Build history of the part. All positions in model axes, mm. A direction names the side the tool comes from. Round coordinates to 2 decimals unless told otherwise and drop trailing zeros. Loops run counter-clockwise (first coordinate to the right, second up) from the corner with the lowest first, then second, coordinate; pieces in that order, holes last.
from build123d import *

# Parameters (mm, degrees)
F0_W     = 88.9
F0_H     = 165.1
F1_DEPTH = 6.35
F2_DEPTH = 25.4
F3_DEPTH = 50.8
F4_SIZE2 = 7.3323484187
F4_SIZE  = 12.7
F5_R     = 6.34999
F6_SIZE2 = 7.3323484187
F6_SIZE  = 12.7
F7_SIZE2 = 7.3323484187
F7_SIZE  = 12.7


# Not quite as in the source:
# - a fillet or chamfer is up to 0.001 mm smaller than in the source, because OpenCascade refuses the exact size


with BuildPart() as f1:
    # F0 (on Top) → F1 (new body)
    with BuildSketch(Plane.XY):
        Rectangle(F0_W, F0_H)
        Polygon((-38.1, 38.1), (-38.1, 76.2), (0, 76.2), (38.1, 76.2), (38.1, -38.1), (38.1, -76.2), (0, -76.2), (-38.1, -76.2), align=None, mode=Mode.SUBTRACT)
    extrude(amount=F1_DEPTH)

    # F0 (on Top) → F2 (join)
    with BuildSketch(Plane.XY):
        with BuildLine():
            Line((38.1, 76.2), (0, 76.2))
            Line((0, 76.2), (0, 50.8))
            ThreePointArc((0, 50.8), (-3.7197438789, 41.8197438789), (-12.7, 38.1))
            Line((-12.7, 38.1), (-38.1, 38.1))
            Line((-38.1, 38.1), (-38.1, -76.2))
            Line((-38.1, -76.2), (0, -76.2))
            Line((0, -76.2), (0, -50.8))
            ThreePointArc((0, -50.8), (3.7197438789, -41.8197438789), (12.7, -38.1))
            Line((12.7, -38.1), (38.1, -38.1))
            Line((38.1, -38.1), (38.1, 76.2))
        make_face()
    extrude(amount=F2_DEPTH)

    # F0 (on Top) → F3 (join)
    with BuildSketch(Plane.XY):
        with BuildLine():
            Line((0, 76.2), (-38.1, 76.2))
            Line((-38.1, 76.2), (-38.1, 38.1))
            Line((-38.1, 38.1), (-12.7, 38.1))
            ThreePointArc((-12.7, 38.1), (-3.7197438789, 41.8197438789), (0, 50.8))
            Line((0, 50.8), (0, 76.2))
        make_face()
        with BuildLine():
            Line((38.1, -76.2), (38.1, -38.1))
            Line((38.1, -38.1), (12.7, -38.1))
            ThreePointArc((12.7, -38.1), (3.7197438789, -41.8197438789), (0, -50.8))
            Line((0, -50.8), (0, -76.2))
            Line((0, -76.2), (38.1, -76.2))
        make_face()
    extrude(amount=F3_DEPTH)

    # F4
    f4_edges = [f1.edges().sort_by_distance(p)[0] for p in [
        (-38.1, -19.05, 25.4),
        (-19.05, -76.2, 25.4),
        (38.1, 19.05, 25.4),
        (19.05, 76.2, 25.4),
    ]]
    f4_side = f1.faces().sort_by_distance((0, 0, 25.4))[0]
    chamfer(f4_edges, length=F4_SIZE, length2=F4_SIZE2, reference=f4_side)

    # F5 (radius 6.35 in the source; OpenCascade refuses exactly that, so slightly less here)
    f5_edges = [f1.edges().sort_by_distance(p)[0] for p in [
        (44.45, 0, 6.35),
        (0, -82.55, 6.35),
        (-44.45, 0, 6.35),
        (0, 82.55, 6.35),
    ]]
    fillet(f5_edges, radius=F5_R)

    # F6
    f6_edges = [f1.edges().sort_by_distance(p)[0] for p in [
        (-19.05, 76.2, 50.8),
        (-38.1, 57.15, 50.8),
    ]]
    chamfer(f6_edges, length=F6_SIZE, length2=F6_SIZE2)

    # F7
    f7_edges = [f1.edges().sort_by_distance(p)[0] for p in [
        (38.1, -57.15, 50.8),
        (19.05, -76.2, 50.8),
    ]]
    chamfer(f7_edges, length=F7_SIZE, length2=F7_SIZE2)


solid = f1.part
(1) Probe line 1 (Z direction, x = -7, y = 5); line 2 (X direction, y = 54, z = 11); line 3 (Y direction, x = 16, z = 33.5). List the from-to ranges inside material, lowest first.
Responses:
line 1: z = 0 to 25.4
line 2: x = -38.1 to 38.1
line 3: y = -76.2 to -38.1
(2) Slice it at D-D on z = 33.5. List the corners of the cut face in (x, y).
Responses:
outline: (-38.1, 38.1) - (-12.7, 38.1) arc R12.7 ccw to (0, 50.8) - (0, 76.2) - (-38.1, 76.2) - close; (0, -76.2) - (38.1, -76.2) - (38.1, -38.1) - (12.7, -38.1) arc R12.7 ccw to (0, -50.8) - close
(3) Which spindle directions (+Z, -Z, +X, -X, +Y, -Y) get a long thin tool onto all of the face, cutting with end or side? Do faces 1 (the face through (15.08, 69.94, 21.68)), 2 (the face through (38.1, -18, 15)), 3 (the face through (-8, 76.2, 18)), 4 (the face through (-31.84, -18.25, 21.68)), 5 (the face through (8, -76.2, 18)). Say none if no direction does.
Responses:
face 1: +Z, +X, +Y
face 2: +Z, +X, +Y, -Y
face 3: +Z, +X, -X, +Y
face 4: +Z, -X, -Y
face 5: +Z, +X, -X, -Y
(4) Pull direction Z, two halves, no side cores. Call faces 6 (the face through (0, 63, 38)), 7 (the face through (-15.08, -69.94, 21.68)): +Z half, -Z half, draft (parallel to the pull), parting line (faces both ways), or undercut.
Responses:
face 6: draft
face 7: +Z half
(5) Slice it at A-A on z = 46.5. List the corners of the cut face in (x, y), plus the area to 3 significant figures.
Responses:
outline: (-33.25, 38.1) - (-12.7, 38.1) arc R12.7 ccw to (0, 50.8) - (0, 71.35) - (-33.25, 71.35) - close; (0, -71.35) - (33.25, -71.35) - (33.25, -38.1) - (12.7, -38.1) arc R12.7 ccw to (0, -50.8) - close
area: 2,140 mm2
(6) Pin check, flat tips, straight feed: P1, Ø20.5, axis at y = 60, z = 38, coming from the +X side; P2, Ø7.5, axis at x = -23.5, z = 40.5, coming from the -Y side; P3, Ø3, axis at x = -25, z = 22, coming from the -Y side. Stop position of each tip, or through.
Responses:
P1: stops at x = 0
P2: stops at y = 38.1
P3: stops at y = -71.99
